Here's how the part is built. I have some questions about the finished solid (model axes, mm). Face numbers are marked on the shaded views. A direction names the side the tool comes from. Give positions to 0.01 mm unless a question says otherwise; leave off trailing zeros. Order: outer loops, then holes, each group sorted by start corner. A loop starts at its lowest first (then second) coordinate and runs counter-clockwise, first axis right, second up. Notation, with made-up numbers: M 53.25,47.5 L 105.25,47.5 A15 ccw 105.25,74.5 Z; hole C -30.75,-35 d8. An arc over 180 degrees is marked long. Use one line per item in the form item = value.
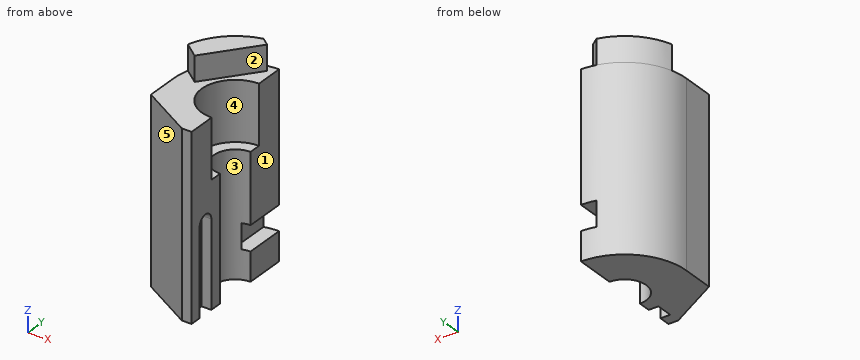
from build123d import *

# Parameters (mm, degrees)
BOSS_EXTRUDE1_DEPTH = 241
CUT_EXTRUDE1_DEPTH  = 78
BOSS_EXTRUDE2_START = 33
BOSS_EXTRUDE2_DEPTH = 33
SKETCH5_W           = 33
SKETCH5_H           = 53.425
CUT_EXTRUDE2_DEPTH  = 19
SKETCH7_W           = 19
SKETCH7_H           = 33
CUT_EXTRUDE3_DEPTH  = 2
CUT_EXTRUDE4_DEPTH  = 13


with BuildPart() as part:
    # Sketch2 → Boss-Extrude1 (new body)
    with BuildSketch(Plane.XY):
        with BuildLine():
            Line((0, -28.575), (0, -82))
            Line((0, -82), (-13, -82))
            Line((-13, -82), (-82, -42.162831426))
            Line((-82, -42.162831426), (-82, 0))
            ThreePointArc((-82, 0), (-57.982756057, 57.982756057), (0, 82))
            Line((0, 82), (0, 28.575))
            ThreePointArc((0, 28.575), (-28.575, 0), (0, -28.575))
        make_face()
    extrude(amount=-BOSS_EXTRUDE1_DEPTH)

    # Sketch3 → Cut-Extrude1 (cut)
    with BuildSketch(Plane.XY):
        with BuildLine():
            Line((0, 44.45), (0, 28.575))
            ThreePointArc((0, 28.575), (-28.575, 0), (0, -28.575))
            Line((0, -28.575), (0, -44.45))
            ThreePointArc((0, -44.45), (-44.45, 0), (0, 44.45))
        make_face()
    extrude(amount=-CUT_EXTRUDE1_DEPTH, mode=Mode.SUBTRACT)

    # Sketch4 → Boss-Extrude2 (add)
    with BuildSketch(Plane.XY.offset(BOSS_EXTRUDE2_START)):
        with BuildLine():
            Line((-18.851828073, 79.803562441), (-8.61759969, 71.807706907))
            Line((-8.61759969, 71.807706907), (-59.101840666, 7.190825111))
            Line((-59.101840666, 7.190825111), (-78.824213609, 22.599631612))
            ThreePointArc((-78.824213609, 22.599631612), (-56.597037955, 59.336121332), (-18.851828073, 79.803562441))
        make_face()
    extrude(amount=-BOSS_EXTRUDE2_DEPTH)

    # Sketch5 → Cut-Extrude2 (cut)
    with BuildSketch(Plane(origin=(0, 0, 0), x_dir=(0, 0, -1), z_dir=(1, 0, 0))):
        with Locations((186.5, 55.2875)):
            Rectangle(SKETCH5_W, SKETCH5_H)
    extrude(amount=-CUT_EXTRUDE2_DEPTH, mode=Mode.SUBTRACT)

    # Sketch7 → Cut-Extrude3 (cut)
    with BuildSketch(Plane(origin=(0, 28.575, 0), x_dir=(1, 0, 0), z_dir=(0, 1, 0))):
        with Locations((-9.5, 186.5)):
            Rectangle(SKETCH7_W, SKETCH7_H)
    extrude(amount=-CUT_EXTRUDE3_DEPTH, mode=Mode.SUBTRACT)

    # Sketch8 → Cut-Extrude4 (cut)
    with BuildSketch(Plane(origin=(0, 0, 0), x_dir=(0, 0, -1), z_dir=(1, 0, 0))):
        with BuildLine():
            Line((241, -45), (127, -45))
            ThreePointArc((127, -45), (116, -56), (127, -67))
            Line((127, -67), (241, -67))
            Line((241, -67), (241, -45))
        make_face()
    extrude(amount=-CUT_EXTRUDE4_DEPTH, mode=Mode.SUBTRACT)


solid = part.part
Q1. On a 3-axis mill with a long thin cutter (end or side, diameter ignored), from which of +Z, -Z, +X, -X, +Y, -Y can I reach the whole of each face in a straight line? I mean the marked faces 4 and 5. Say none if no direction works.
Found:
face_4 = +Z, +X
face_5 = +Z, -Z, -X, -Y
Q2. I need wall thicknesses on L1, parallel to Z at x = -4.5, y = 38; L2, parallel to Z at x = -67, y = -13.5; L3, parallel to Y at x = -12, z = -174 (3 decimals). Which ranges of each line are inside material? Lowest first, please.
Found:
L1 = -241 to -203, -170 to -78
L2 = -241 to 0
L3 = -82 to -67, -45 to -25.933, 25.933 to 26.575
Q3. I want a section at C-C on y = 36. Write out the boundary of the cut face in (x, z).
Found:
outline = M -73.67,-241 L 0,-241 L 0,-203 L -19,-203 L -19,-170 L 0,-170 L 0,-78 L -26.07,-78 L -26.07,0 L -36.59,0 L -36.59,33 L -73.67,33 Z
Q4. Thinking about a two-plate mould opening in Y: for the marked faces 1, 2 and 3, which applies, +Y half, -Y half, draft (parallel to the pull), parting line (faces both ways), or undercut?
Found:
face_1 = draft
face_2 = -Y half
face_3 = undercut
Q5. I want a section at B-B on x = -72. Write out the boundary of the cut face in (y, z), then the cut area to 3 significant figures.
Found:
outline = M -47.94,-241 L 39.24,-241 L 39.24,33 L 17.27,33 L 17.27,0 L -47.94,0 Z
area = 21,700 mm²
Q6. I want a section at D-D on z = -81. Write out the boundary of the cut face in (x, y) (3 decimals), then the cut area to 3 significant figures.
Found:
outline = M -82,-42.163 L -13,-82 L 0,-82 L 0,-28.575 A28.575 cw 0,28.575 L 0,82 A82 ccw -82,0 Z
area = 9,350 mm²
Q7. I want a section at A-A on z = -198. Write out the boundary of the cut face in (x, y) (3 decimals), then the cut area to 3 significant figures.
Found:
outline = M -82,-42.163 L -13,-82 L 0,-82 L 0,-67 L -13,-67 L -13,-45 L 0,-45 L 0,-28.575 A28.575 cw -10.502,26.575 L -19,26.575 L -19,79.768 A82 ccw -82,0 Z
area = 8,040 mm²
Q8. I'm going to push flat-ended pins straight in: pin 1 Ø21 at (x, y) = (-5.5, 42.5) entering from +Z; pin 2 Ø1.5 at (x, y) = (-8.5, 40) entering from +Z; pin 3 Ø7 at (x, z) = (-16, -189) entering from +Y. Where does each tip first touch, or does it pass through?
Found:
pin_1 = 0
pin_2 = -78
pin_3 = 79.77
